```python
from build123d import *

# Parameters (mm, degrees)
SKETCH1_R           = 45
BOSS_EXTRUDE1_DEPTH = 40
SKETCH2_R           = 50
BOSS_EXTRUDE2_DEPTH = 5
BOSS_EXTRUDE3_START = 5
SKETCH3_R           = 50
BOSS_EXTRUDE3_DEPTH = 5
SKETCH4_R           = 35
CUT_EXTRUDE1_DEPTH  = 20
CUT_EXTRUDE2_START  = -20
SKETCH5_R           = 35
CUT_EXTRUDE2_DEPTH  = 20
SKETCH6_R           = 6
CUT_EXTRUDE3_DEPTH  = 20
CUT_EXTRUDE4_DEPTH  = 10


with BuildPart() as part:
    # Sketch1 → Boss-Extrude1 (new body)
    with BuildSketch(Plane.XY):
        Circle(SKETCH1_R)
    extrude(amount=BOSS_EXTRUDE1_DEPTH)

    # Sketch2 → Boss-Extrude2 (add)
    with BuildSketch(Plane.XY.offset(40)):
        Circle(SKETCH2_R)
    extrude(amount=BOSS_EXTRUDE2_DEPTH)

    # Sketch3 → Boss-Extrude3 (add)
    with BuildSketch(Plane(origin=(0, 0, 0), x_dir=(-1, 0, 0), z_dir=(0, 0, -1)).offset(BOSS_EXTRUDE3_START)):
        with Locations(Location((0, 0, 0), (0, 0, 180))):
            Circle(SKETCH3_R)
    extrude(amount=-BOSS_EXTRUDE3_DEPTH)

    # Sketch4 → Cut-Extrude1 (cut)
    with BuildSketch(Plane.XY.offset(45)):
        Circle(SKETCH4_R)
    extrude(amount=-CUT_EXTRUDE1_DEPTH, mode=Mode.SUBTRACT)

    # Sketch5 → Cut-Extrude2 (cut)
    with BuildSketch(Plane(origin=(0, 0, -5), x_dir=(-1, 0, 0), z_dir=(0, 0, -1)).offset(CUT_EXTRUDE2_START)):
        with Locations(Location((0, 0, 0), (0, 0, 180))):
            Circle(SKETCH5_R)
    extrude(amount=CUT_EXTRUDE2_DEPTH, mode=Mode.SUBTRACT)

    # Sketch6 → Cut-Extrude3 (cut)
    with BuildSketch(Plane.XY.offset(25)):
        Circle(SKETCH6_R)
    extrude(amount=-CUT_EXTRUDE3_DEPTH, mode=Mode.SUBTRACT)

    # Sketch7 → Cut-Extrude4 (cut)
    with BuildSketch(Plane.XY.offset(25)):
        Polygon((-20, -0.07309958), (-20, -2.57309958), (-30, -2.57309958), (-30, -0.07309958), (-30, 2.42690042), (-20, 2.42690042), align=None)
    extrude(amount=-CUT_EXTRUDE4_DEPTH, mode=Mode.SUBTRACT)


solid = part.part
```
Here's how the part is built. I have some questions about the finished solid (model axes, mm). A direction names the side the tool comes from. Coordinates: 2 decimals unless noted, no trailing zeros. Order: outer loops, then holes, each group sorted by start corner. A loop starts at its lowest first (then second) coordinate and runs counter-clockwise, first axis right, second up. Notation, with made-up numbers: (8.5, -28) -> (62.5, -28) arc R17 ccw to (62.5, -14) -> close; hole circle Ø8 at (-16, 27). An arc over 180 degrees is marked (long way). Return JSON: item names as keys, results as strings.
1) If we section it at A-A on y = 0: List the corners of the cut face in (x, z) for me, plus the area to 3 significant figures.
Conclusion:
{"outline": "(-50, -5) -> (-35, -5) -> (-35, 15) -> (-30, 15) -> (-30, 25) -> (-35, 25) -> (-35, 45) -> (-50, 45) -> (-50, 40) -> (-45, 40) -> (-45, 0) -> (-50, 0) -> close; (-20, 15) -> (-6, 15) -> (-6, 25) -> (-20, 25) -> close; (6, 15) -> (35, 15) -> (35, -5) -> (50, -5) -> (50, 0) -> (45, 0) -> (45, 40) -> (50, 40) -> (50, 45) -> (35, 45) -> (35, 25) -> (6, 25) -> close", "area": "1,580 mm²"}
2) If I drill on probe 1 along Y at (x, z) = (0, 20); probe 2 along Y at (x, z) = (0, 38.5); probe 3 along Z at (x, y) = (-33.5, -36.5), over which ranges is the centre line in solid material (lowest first)?
Conclusion:
{"probe 1": "y = -45 to -6, 6 to 45", "probe 2": "y = -45 to -35, 35 to 45", "probe 3": "z = -5 to 0, 40 to 45"}
3) If we section it at C-C on z = 23: List the corners of the cut face in (x, y) for me.
Conclusion:
{"outline": "circle Ø90 at (0, 0); hole (-30, -2.57) -> (-20, -2.57) -> (-20, 2.43) -> (-30, 2.43) -> close; hole circle Ø12 at (0, 0)"}
4) On a 3-axis mill with a long thin cutter (end or side, diameter ignored), from which of +Z, -Z, +X, -X, +Y, -Y can I reach the whole of each face in a straight line? I mean faces 1 (the flat face through (7, 0, 15)), 2 (the cylindrical face through (-28, -21, 35)), 3 (the flat face through (-30, 0, 20)), 4 (the flat face through (-41, -19, 0)). Say none if no direction works.
Conclusion:
{"face 1": "-Z", "face 2": "+Z", "face 3": "+Z, -Z", "face 4": "none"}
5) If we section it at D-D on x = -43: List the corners of the cut face in (y, z) for me.
Conclusion:
{"outline": "(-25.51, -5) -> (25.51, -5) -> (25.51, 0) -> (13.27, 0) -> (13.27, 40) -> (25.51, 40) -> (25.51, 45) -> (-25.51, 45) -> (-25.51, 40) -> (-13.27, 40) -> (-13.27, 0) -> (-25.51, 0) -> close"}
6) I'm going to push flat-ended pins straight in: P1, Ø2, axis at x = 33, z = 13.5, coming from the +Y side; P2, Ø8, axis at y = -21, z = 19, coming from the -X side; P3, Ø8, axis at x = 24.5, y = -7, coming from the +Z side. Where does each tip first touch, or does it pass through?
Conclusion:
{"P1": "stops at y = 31.64", "P2": "stops at x = -41.67", "P3": "stops at z = 25"}
7) Thinking about a two-plate mould opening in Y: for faces 5 (the flat face through (-41, 19, 40)), 6 (the flat face through (-20, 0, 20)), 7 (the cylindrical face through (20.765, -39.923, 19.72)), which applies, +Y half, -Y half, draft (parallel to the pull), parting line (faces both ways), or undercut?
Conclusion:
{"face 5": "draft", "face 6": "undercut", "face 7": "parting line"}
8) If we section it at B-B on x = 0: List the corners of the cut face in (y, z) for me, plus the area to 3 significant figures.
Conclusion:
{"outline": "(-50, -5) -> (-35, -5) -> (-35, 15) -> (-6, 15) -> (-6, 25) -> (-35, 25) -> (-35, 45) -> (-50, 45) -> (-50, 40) -> (-45, 40) -> (-45, 0) -> (-50, 0) -> close; (6, 15) -> (35, 15) -> (35, -5) -> (50, -5) -> (50, 0) -> (45, 0) -> (45, 40) -> (50, 40) -> (50, 45) -> (35, 45) -> (35, 25) -> (6, 25) -> close", "area": "1,680 mm²"}
